```python
from build123d import *

# Parameters (mm, degrees)
SKETCH1_W           = 105
SKETCH1_H           = 65
BOSS_EXTRUDE1_DEPTH = 45
SKETCH2_R           = 5
BOSS_EXTRUDE2_DEPTH = 5
SKETCH3_R           = 4.5
BOSS_EXTRUDE3_DEPTH = 20
SKETCH4_R           = 5
BOSS_EXTRUDE4_DEPTH = 5
SKETCH5_R           = 4.5
BOSS_EXTRUDE5_DEPTH = 20


with BuildPart() as part:
    # Sketch1 → Boss-Extrude1 (new body)
    with BuildSketch(Plane.XY):
        Rectangle(SKETCH1_W, SKETCH1_H)
    extrude(amount=BOSS_EXTRUDE1_DEPTH)

    # Sketch2 → Boss-Extrude2 (add)
    with BuildSketch(Plane.ZY.offset(52.5)):
        with Locations((9.080491803, 21.421132833)):
            Circle(SKETCH2_R)
    extrude(amount=BOSS_EXTRUDE2_DEPTH)

    # Sketch3 → Boss-Extrude3 (add)
    with BuildSketch(Plane.ZY.offset(57.5)):
        with Locations((9.080491803, 21.421132833)):
            Circle(SKETCH3_R)
    extrude(amount=BOSS_EXTRUDE3_DEPTH)

    # Sketch4 → Boss-Extrude4 (add)
    with BuildSketch(Plane(origin=(52.5, 0, 0), x_dir=(0, 0, -1), z_dir=(1, 0, 0))):
        with Locations((-11.51313285, 24.423590695)):
            Circle(SKETCH4_R)
    extrude(amount=BOSS_EXTRUDE4_DEPTH)

    # Sketch5 → Boss-Extrude5 (add)
    with BuildSketch(Plane(origin=(57.5, 0, 0), x_dir=(0, 0, -1), z_dir=(1, 0, 0))):
        with Locations((-11.51313285, 24.423590695)):
            Circle(SKETCH5_R)
    extrude(amount=BOSS_EXTRUDE5_DEPTH)


solid = part.part
```
The listing builds one solid part. Answer for the finished solid, in the listing's coordinates (mm). A direction names the side the tool comes from. Coordinates: 2 decimals unless noted, no trailing zeros. Write each loop counter-clockwise with the first axis right and the second up, starting at its lowest first coordinate (ties: lowest second). Pieces come first, ordered by that corner, then holes.
Q1. Given P1, Ø4, axis at y = 20, z = 26, coming from the -X side; P2, Ø5, axis at y = -23.5, z = 31.5, coming from the +X side; P3, Ø5, axis at x = 25.5, y = 7.5, coming from the -Z side; P4, Ø3, axis at x = 59, z = 18.5, coming from the -Y side, each flat-ended and moving along its own axis, determine where each tip first touches the part or whether it passes through.
Returned:
P1: stops at x = -52.5
P2: stops at x = 52.5
P3: stops at z = 0
P4: passes through
Q2. Section C-C, the plane x = -67.5 is taken. Write down the section's boundary in (y, z).
Returned:
outline: circle Ø9 at (21.42, 9.08)
Q3. Section B-B, the plane y = -9.5 is taken. Write down the section's boundary in (x, z).
Returned:
outline: (-52.5, 0) - (52.5, 0) - (52.5, 45) - (-52.5, 45) - close
Q4. Section A-A, the plane z = 30.5 is taken. Write down the section's boundary in (x, y).
Returned:
outline: (-52.5, -32.5) - (52.5, -32.5) - (52.5, 32.5) - (-52.5, 32.5) - close
Q5. Section D-D, the plane x = 55.5 is taken. Write down the section's boundary in (y, z).
Returned:
outline: circle Ø10 at (24.42, 11.51)
Q6. Find the intervals of material crossed by line 1 along X through (y, z) = (-27, 9.5); line 2 along Z through (x, y) = (66, 25); line 3 along Y through (x, z) = (59, 14), in increasing order.
Returned:
line 1: x = -52.5 to 52.5
line 2: z = 7.05 to 15.98
line 3: y = 20.67 to 28.17
Q7. Which of the six approach directions +Z, -Z, +X, -X, +Y, -Y give full straight-line access (tool end or side, diameter ignored) to faces 1 (the cylindrical face through (-54.96, 16.54, 8)), 2 (the flat face through (77.5, 24, 12)), 3 (the cylindrical face through (54.96, 21.38, 15.48))?
Returned:
face 1: -X
face 2: +Z, -Z, +X, +Y, -Y
face 3: +X
